Read the model definition and answer for the solid it produces. Units are mm, in the model's axes. Face numbers are marked on the shaded views. A direction names the side the tool comes from. Round coordinates to 2 decimals unless told otherwise and drop trailing zeros. Write each loop counter-clockwise with the first axis right and the second up, starting at its lowest first coordinate (ties: lowest second). Pieces come first, ordered by that corner, then holes. Notation, with made-up numbers: (77.25, 2) -> (101.25, 2) arc R18 cw to (101.25, 15) -> close; hole circle Ø3 at (2.5, 53). An arc over 180 degrees is marked (long way). Return JSON: item names as keys, results as strings. Group by question number.
(1) A cutting plane is placed at A-A on x = -5.25. Give the vertices of the cut face in (y, z), then the cut area to 3 significant figures.
(2) A cutting plane is placed at D-D on x = -17. Give the vertices of the cut face in (y, z).
(3) A cutting plane is placed at C-C on z = 11.5. Give the vertices of the cut face in (x, y) (3 decimals).
(4) Straight lines are drawn through the part: line 1 (Z direction, x = -9.75, y = 16.75); line 2 (Y direction, x = -6, z = 8); line 3 (X direction, y = 4.25, z = 8.5). For each, find the intervals that lie inside material, in ascending order.
(5) A cutting plane is placed at B-B on y = 5.25. Give the vertices of the cut face in (x, z), then the cut area to 3 significant figures.
(6) For the marked faces 4 and 5, determine the directions among +Z, -Z, +X, -X, +Y, -Y from which every point of the face is accessible in a straight line to the end or side of a thin tool.
(7) Given pin 1 (3.5 mm diameter, centred on y = 13, z = 10, fed in from -X); pin 2 (1.9 mm diameter, centred on x = -7, z = 11.5, fed in from +Y); pin 3 (9 mm diameter, centred on x = -9.5, y = 11, fed in from +Z), each flat-ended and moving along its own axis, determine where each tip first touches the part or whether it passes through.
(8) The mould has two halves that part along X. Classify the marked faces 1, 2 and 3: released by +X, released by -X, zero draft, split by the parting line, or undercut.
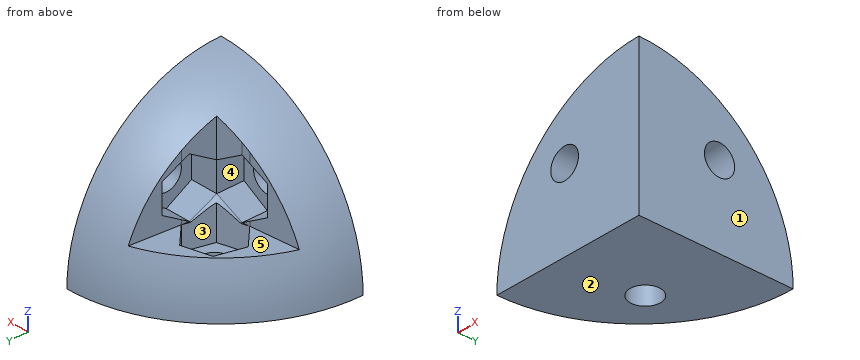
```python
from build123d import *

# Parameters (mm, degrees)
REVOLVE1_ANGLE     = 90
SKETCH2_R          = 2.15
EXTRUDE1_DEPTH     = 39.105117767
EXTRUDE2_START     = 4
EXTRUDE2_DEPTH     = 35.105117767
EXTRUDE4_START     = -4
EXTRUDE4_DEPTH     = 35.105117767
CUT_REVOLVE1_START = 7.343078062
CUT_REVOLVE1_DEPTH = 11.608966683
EXTRUDE5_DEPTH     = 36.944401511


# Read off the part's stored shape, not the designer's step: Cut-Revolve1
with BuildPart() as part:
    # Sketch1 → Revolve1 (revolve)
    with BuildSketch(Plane(origin=(0, 0, 0), x_dir=(0, 0, -1), z_dir=(1, 0, 0))):
        with BuildLine():
            Line((0, 0), (0, 22))
            ThreePointArc((0, 22), (-15.556349186, 15.556349186), (-22, 0))
            Line((-22, 0), (0, 0))
        make_face()
    revolve(axis=Axis((0, 0, 0), (0, -1, 0)), revolution_arc=REVOLVE1_ANGLE)

    # Sketch2 → Extrude1 (cut, through all)
    with BuildSketch(Plane(origin=(0, 0, 0), x_dir=(1, 0, 0), z_dir=(0, 1, 0))):
        with Locations(Location((-11.5, -11.5, 0), (0, 0, 225))):
            Circle(SKETCH2_R)
    extrude1 = extrude(amount=EXTRUDE1_DEPTH, mode=Mode.SUBTRACT)

    # Sketch4 → Extrude2 (cut, through all)
    with BuildSketch(Plane(origin=(0, 0, 0), x_dir=(1, 0, 0), z_dir=(0, 1, 0)).offset(EXTRUDE2_START)):
        Polygon((-7.9, -9.421539031), (-11.5, -7.343078062), (-15.1, -9.421539031), (-15.1, -13.578460969), (-11.5, -15.656921938), (-7.9, -13.578460969), align=None)
    extrude2 = extrude(amount=EXTRUDE2_DEPTH, mode=Mode.SUBTRACT)

    # Mirror1: Extrude1 across plane
    add(extrude1.mirror(Plane(origin=(0, 0, 0), x_dir=(2.468850131082266e-15, 0.7071067811865478, 0.7071067811865472), z_dir=(2.4688501310822653e-15, 0.7071067811865475, -0.7071067811865477))), mode=Mode.SUBTRACT)

    # Mirror5: Extrude1, Extrude2 across plane
    add(extrude1.mirror(Plane(origin=(0, 0, 0), x_dir=(0, 0, 1), z_dir=(-0.7071067811865475, -0.7071067811865477, 0))), mode=Mode.SUBTRACT)
    add(extrude2.mirror(Plane(origin=(0, 0, 0), x_dir=(0, 0, 1), z_dir=(-0.7071067811865475, -0.7071067811865477, 0))), mode=Mode.SUBTRACT)

    # Sketch9 → Extrude4 (cut, through all)
    with BuildSketch(Plane(origin=(0, 0, 0), x_dir=(-1, 0, 0), z_dir=(0, 0, -1)).offset(EXTRUDE4_START)):
        Polygon((8.560612309, 8.560612309), (12.575890567, 7.484721742), (15.515278258, 10.424109433), (14.439387691, 14.439387691), (10.424109433, 15.515278258), (7.484721742, 12.575890567), align=None)
    extrude(amount=-EXTRUDE4_DEPTH, mode=Mode.SUBTRACT)

    # Cut-Revolve1 outline → Cut-Revolve1 (cut)
    with BuildSketch(Plane.XY.offset(CUT_REVOLVE1_START)):
        Polygon((-11.5, 7.58027444), (-7.9, 7.9), (-7.484721742, 12.575890567), (-8.560612309, 8.560612309), (-12.575890567, 7.484721742), align=None)
        Polygon((-7.484721742, 12.575890567), (-6.863589335, 19.569628152), (-6.736554213, 21), (-21, 21), (-21, 6.736554212), (-19.569628152, 6.863589334), (-12.575890567, 7.484721742), (-15.515278258, 10.424109433), (-14.439387691, 14.439387691), (-10.424109433, 15.515278258), align=None)
    extrude(amount=CUT_REVOLVE1_DEPTH, mode=Mode.SUBTRACT)

    # Sketch11 → Revolve4 (revolve)
    with BuildSketch(Plane(origin=(-0.757954206, 8.534304053, 0), x_dir=(0.9960793346659582, 0.08846445077782496, 0), z_dir=(-0.08846445077782496, 0.9960793346659582, 0))):
        Polygon((-7.170157583, -9.421539031), (-7.170157583, -7.343078062), (-10.784327534, -7.343078062), align=None)
    revolve(axis=Axis((-7.9, 7.9, 9.421539031), (0, 0, -1)))

    # Sketch12 → Extrude5 (cut, through all)
    with BuildSketch(Plane.XY.offset(4)):
        Polygon((-8.560612309, 8.560612309), (-7.484721742, 12.575890567), (-10.424109433, 15.515278258), (-14.439387691, 14.439387691), (-15.515278258, 10.424109433), (-12.575890567, 7.484721742), align=None)
    extrude(amount=EXTRUDE5_DEPTH, mode=Mode.SUBTRACT)


solid = part.part
```
Checks:
{
 "1": {"outline": "(0, 0) -> (21.36, 0) arc R21.36 ccw to (0, 21.36) -> close; hole (7.9, 9.42) -> (11.5, 7.34) -> (15.1, 9.42) -> (15.1, 13.58) -> (11.5, 15.66) -> (7.9, 13.58) -> close", "area": "314 mm^2"},
 "2": {"outline": "(0, 0) -> (13.96, 0) arc R13.96 ccw to (11.88, 7.34) -> (7.09, 7.34) -> (7.09, 12.03) arc R13.96 ccw to (0, 13.96) -> close"},
 "3": {"outline": "(-18.755, 0) -> (-13.65, 0) -> (-13.65, 4) -> (-15.1, 4) -> (-15.1, 7.261) -> (-17.376, 7.058) arc R18.755 ccw to start; (-9.35, 0) -> (0, 0) -> (0, 9.35) -> (-4, 9.35) -> (-4, 7.9) -> (-7.9, 7.9) -> (-7.9, 4) -> (-9.35, 4) -> close; (-7.261, 15.1) -> (-4, 15.1) -> (-4, 13.65) -> (0, 13.65) -> (0, 18.755) arc R18.755 ccw to (-7.058, 17.376) -> close"},
 "4": {"line 1": "z = 0 to 7.34", "line 2": "y = 0 to 10.36, 12.64 to 19.6", "line 3": "x = -19.84 to -13.5, -9.5 to 0"},
 "5": {"outline": "(-21.36, 0) -> (0, 0) -> (0, 21.36) arc R21.36 ccw to start; hole (-15.1, 9.42) -> (-11.5, 7.34) -> (-7.9, 9.42) -> (-7.9, 13.58) -> (-11.5, 15.66) -> (-15.1, 13.58) -> close", "area": "314 mm^2"},
 "6": {"face 4": "+Y", "face 5": "+Z, -X, +Y"},
 "7": {"pin 1": "stops at x = -7.44", "pin 2": "stops at y = 18.09", "pin 3": "stops at z = 19.58"},
 "8": {"face 1": "released by +X", "face 2": "zero draft", "face 3": "undercut"}
}
